```python
from build123d import *

# Parameters (mm, degrees)
SKETCH1_R           = 2
BOSS_EXTRUDE1_DEPTH = 5
FILLET1_R           = 50
FILLET2_R           = 8
FILLET3_R           = 3.75
FILLET4_R           = 3.75


with BuildPart() as part:
    # Sketch1 → Boss-Extrude1 (new, symmetric)
    with BuildSketch(Plane.XY):
        Polygon((0, 0), (-7.5, 0), (-7.5, 8), (-7.5, 10.5), (44.5, 10.5), (44.5, 8), (44.5, 0), (37, 0), (37, 5), (12.5, 8), (0, 5), align=None)
        with Locations((-3.75, 3)):
            Circle(SKETCH1_R, mode=Mode.SUBTRACT)
        with Locations((40.75, 3)):
            Circle(SKETCH1_R, mode=Mode.SUBTRACT)
    extrude(amount=BOSS_EXTRUDE1_DEPTH, both=True)

    # Fillet1
    fillet1_edges = [part.edges().sort_by_distance(p)[0] for p in [
        (12.5, 8, 0),
    ]]
    fillet(fillet1_edges, radius=FILLET1_R)

    # Fillet2
    fillet2_edges = [part.edges().sort_by_distance(p)[0] for p in [
        (-7.5, 10.5, 0),
        (44.5, 10.5, 0),
    ]]
    fillet(fillet2_edges, radius=FILLET2_R)

    # Fillet3
    # the kernel refuses this fillet: 3.75 mm, written as the material it takes off along each edge
    with BuildSketch(Plane(origin=(44.5, 0, 17.164560514), x_dir=(-0.0727207133761252, 0.997352343881573, 0), z_dir=(0, 0, -1))) as fillet3_piece_1:
        with BuildLine():
            CenterArc((4.026444062, -3.654851704), FILLET3_R, 77.065635914, 107.104635177)
            Line((0.286372773, -3.927554379), (-0.087634356, -3.954824646))
            Line((-0.087634356, -3.954824646), (-0.374007129, -0.027270268))
            Line((-0.374007129, -0.027270268), (-0.027270268, 0.374007129))
            ThreePointArc((-0.027270268, 0.374007129), (2.466110592, 0.555808912), (4.94976222, 0.36548517))
            Line((4.94976222, 0.36548517), (4.865824206, 0))
        make_face()
    extrude(amount=34.329121028, mode=Mode.SUBTRACT)
    with BuildSketch(Plane(origin=(37, 0, 14.375), x_dir=(1, 0, 0), z_dir=(0, 0, -1)), Plane(origin=(0, 0, -14.375), x_dir=(-1, 0, 0), z_dir=(0, 0, 1))) as fillet3_piece_2:
        with BuildLine():
            CenterArc((FILLET3_R, -FILLET3_R), FILLET3_R, 90, 90)
            Line((0, -FILLET3_R), (0, 0))
            Line((0, 0), (FILLET3_R, 0))
        make_face()
    extrude(amount=28.75, mode=Mode.SUBTRACT)
    with BuildSketch(Plane(origin=(-7.5, 0, 17.164560514), x_dir=(0.07272071337612518, 0.997352343881573, 0), z_dir=(0, 0, -1))) as fillet3_piece_3:
        with BuildLine():
            CenterArc((4.026444062, 3.654851704), FILLET3_R, 175.829728909, 107.104635177)
            Line((0.286372773, 3.927554379), (-0.087634356, 3.954824646))
            Line((-0.087634356, 3.954824646), (-0.374007129, 0.027270268))
            Line((-0.374007129, 0.027270268), (-0.027270268, -0.374007129))
            ThreePointArc((-0.027270268, -0.374007129), (2.466110592, -0.555808912), (4.94976222, -0.36548517))
            Line((4.94976222, -0.36548517), (4.865824206, 0))
        make_face()
    extrude(amount=34.329121028, mode=Mode.SUBTRACT)

    # Fillet4
    fillet4_edges = [part.edges().sort_by_distance(p)[0] for p in [
        (0, 5, 0),
        (37, 5, 0),
    ]]
    fillet(fillet4_edges, radius=FILLET4_R)


solid = part.part
```
Verification items for the finished model (mm, model axes). A direction names the side the tool comes from. Give positions to 0.01 mm unless a question says otherwise; leave off trailing zeros. Write each loop counter-clockwise with the first axis right and the second up, starting at its lowest first coordinate (ties: lowest second). Pieces come first, ordered by that corner, then holes. Notation, with made-up numbers: M -16.5,-6 L 20.5,-6 A12 ccw 20.5,13 Z; hole C 58,-13.5 d6. An arc over 180 degrees is marked long. One line per question, with ' | ' between items.
1) Section check D-D on y = 9.25. Enter the section's corners in (x, z), plus the area to 3 significant figures.
Result:
outline: M -3.79,-5 L 40.79,-5 L 40.79,5 L -3.79,5 Z | area: 446 mm2
2) Thickness scan on line 1 along X through (y, z) = (3.5, -4); line 2 along X through (y, z) = (2.25, -3.5); line 3 along Y through (x, z) = (40.75, 2.25). Record the ranges inside material, lowest first. Write a range as [from, to].
Result:
line 1: x = [-7.3, -5.69], [-1.81, 0.11], [36.81, 38.81], [42.69, 44.3] | line 2: x = [-7, -5.6], [-1.9, -0.31], [37.31, 38.9], [42.6, 44] | line 3: y = [0, 1], [5, 9.28]
3) Section check B-B on z = 1.5. State how many separate pieces and enclosed holes the cut face has, plus the area to 3 significant figures.
Result:
separate pieces: 1 | enclosed holes: 2 | area: 247 mm2
4) Section check C-C on x = 19. Enter the section's corners in (y, z).
Result:
outline: M 7.14,-5 L 10.5,-5 L 10.5,5 L 7.14,5 Z
5) Mould release check, pull along X, two halves, no side actions. Record for faces 1 (the cylindrical face through (-6.578, 1.521, 0.07)), 2 (the cylindrical face through (43.634, 1.6, 0.07)), 3 (the cylindrical face through (-1.42, 0.81, -0.07)): released by +X, released by -X, zero draft, split by the parting line, or undercut.
Result:
face 1: released by -X | face 2: released by +X | face 3: undercut
6) Set-up check for faces 4 (the cylindrical face through (41.195, 8.977, -0.07)), 5 (the flat face through (3.2, 5.77, 0.07)): record each of +Z, -Z, +X, -X, +Y, -Y from which the full face is reachable in a straight line by a thin tool's end or side.
Result:
face 4: +Z, -Z, +X, +Y | face 5: +Z, -Z, -Y
7) Section check A-A on y = 1.75. Enter the section's corners in (x, z).
Result:
outline: M -6.73,-5 L -5.31,-5 L -5.31,5 L -6.73,5 Z; M -2.19,-5 L -0.58,-5 L -0.58,5 L -2.19,5 Z; M 37.58,-5 L 39.19,-5 L 39.19,5 L 37.58,5 Z; M 42.31,-5 L 43.73,-5 L 43.73,5 L 42.31,5 Z
8) Gauge pin test, flat ends, axial feed: pin 1 Ø3 at (x, y) = (40.75, 3) entering from -Z; pin 2 Ø6 at (x, z) = (37.5, 2) entering from -Y; pin 3 Ø1.5 at (y, z) = (8, -3) entering from +X; pin 4 Ø1.5 at (x, z) = (8.5, 1.5) entering from -Y. Record the tip position at first contact, or that the pin passes through.
Result:
pin 1: passes through | pin 2: stops at y = 0.01 | pin 3: stops at x = 42.94 | pin 4: stops at y = 6.69
